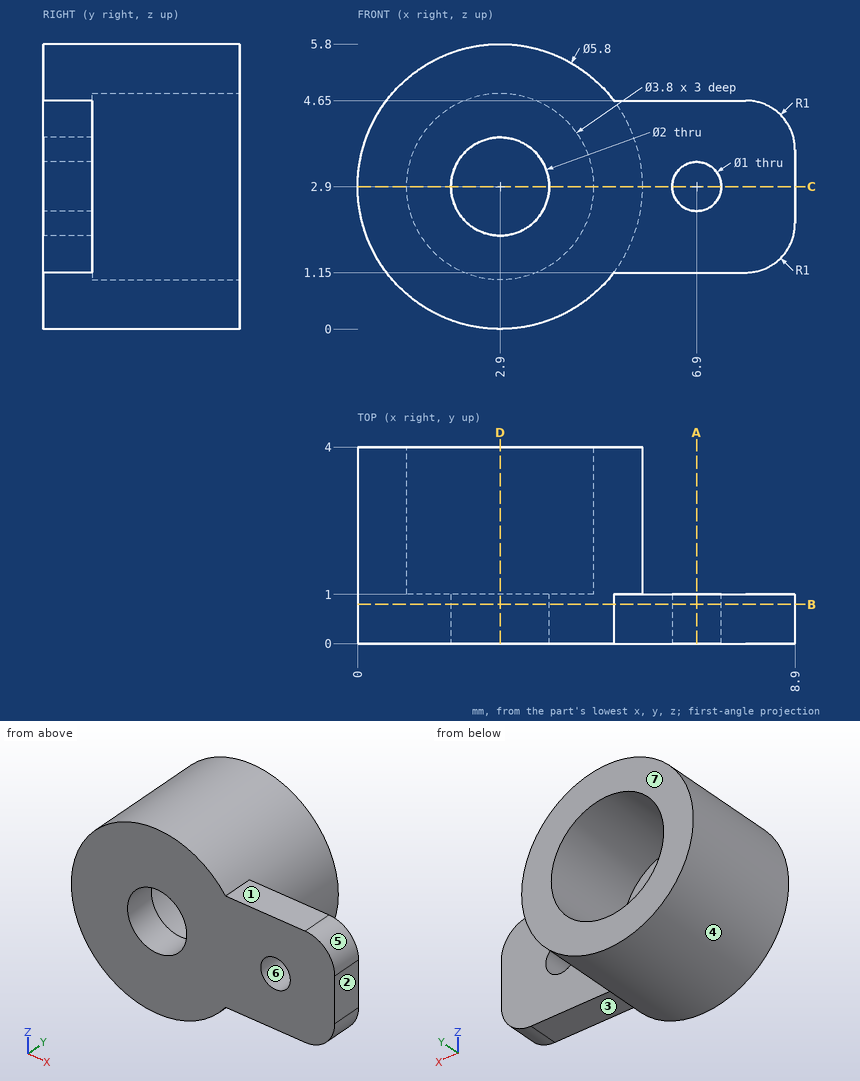
Study the drawing (mm; zero at the part's minimum x, y, z) and answer. A direction names the side the tool comes from. Give positions to 0.01 mm unless a question says otherwise; leave off trailing zeros. Order: outer loops, then holes, each group sorted by start corner. A loop starts at its lowest first (then second) coordinate and runs counter-clockwise, first axis right, second up. Notation, with made-up numbers: M -11.75,79.25 L 17.25,79.25 A20 cw 17.25,92.25 Z; hole C 19.25,24 d5. An arc over 180 degrees is marked long. Put each result on its own line as item: value. Start each with the question number.
Item 1: Which of the six approach directions +Z, -Z, +X, -X, +Y, -Y give full straight-line access (tool end or side, diameter ignored) to the marked faces 1, 2, 3 and 4?
Item 2: The part is cut by section D-D, the plane x = 2.9. Determine the outline of the cut face in (y, z).
Item 3: The part is cut by section A-A, the plane x = 6.9. Determine the outline of the cut face in (y, z).
Item 4: The part is cut by section C-C, the plane z = 2.9. Determine the outline of the cut face in (x, y), and give its area (3 significant figures).
Item 5: Flat-ended cylindrical pins translate along their axes: P1, Ø0.8, axis at x = 6, y = 0.5, coming from the -Z side; P2, Ø2.5, axis at x = 2.9, z = 2.9, coming from the +Y side. Find the tip coordinate at first contact, or state that the pin passes through.
Item 6: The part is cut by section B-B, the plane y = 0.8. Determine the outline of the cut face in (x, z), and give its area (3 significant figures).
Item 7: Find the intervals of material crossed by line 1 along X through (y, z) = (0.75, 2.9); line 2 along X through (y, z) = (3.15, 2.9); line 3 along Z through (x, y) = (2.9, 0.5), in increasing order.
Item 8: For a pull along X with two mould halves and no side action, classify the marked faces 5, 6 and 7 as +X half, -X half, draft (parallel to the pull), parting line (faces both ways), or undercut.
Answer key:
1. face 1: +Z, +X, +Y, -Y
1. face 2: +Z, -Z, +X, +Y, -Y
1. face 3: -Z, +X, +Y, -Y
1. face 4: +Y
2. outline: M 0,0 L 4,0 L 4,1 L 1,1 L 1,1.9 L 0,1.9 Z; M 0,3.9 L 1,3.9 L 1,4.8 L 4,4.8 L 4,5.8 L 0,5.8 Z
3. outline: M 0,1.15 L 1,1.15 L 1,2.4 L 0,2.4 Z; M 0,3.4 L 1,3.4 L 1,4.65 L 0,4.65 Z
4. outline: M 0,0 L 1.9,0 L 1.9,1 L 1,1 L 1,4 L 0,4 Z; M 3.9,0 L 6.4,0 L 6.4,1 L 5.8,1 L 5.8,4 L 4.8,4 L 4.8,1 L 3.9,1 Z; M 7.4,0 L 8.9,0 L 8.9,1 L 7.4,1 Z
4. area: 11.9 mm²
5. P1: stops at z = 1.15
5. P2: stops at y = 1
6. outline: M 5.21,1.15 L 7.9,1.15 A1 ccw 8.9,2.15 L 8.9,3.65 A1 ccw 7.9,4.65 L 5.21,4.65 A2.9 ccw long Z; hole C 2.9,2.9 d2; hole C 6.9,2.9 d1
6. area: 33.6 mm²
7. line 1: x = 0 to 1.9, 3.9 to 6.4, 7.4 to 8.9
7. line 2: x = 0 to 1, 4.8 to 5.8
7. line 3: z = 0 to 1.9, 3.9 to 5.8
8. face 5: +X half
8. face 6: undercut
8. face 7: draft
